from build123d import *

# Parameters (mm, degrees)
F0_W     = 114.3
F0_H     = 88.9
F1_DEPTH = 152.4
F3_R     = 38.1
F4_R     = 12.7
F5_DEPTH = 114.301
F6_R     = 6.35
F7_DEPTH = 38.1
F2_W     = 19.05
F2_H     = 88.9
F2_W_2   = 25.4
F8_DEPTH = 88.901


with BuildPart() as f1:
    # F0 (on Top) → F1 (new body)
    with BuildSketch(Plane.XY):
        Rectangle(F0_W, F0_H)
    extrude(amount=F1_DEPTH)

    # F3
    f3_edges = [f1.edges().sort_by_distance(p)[0] for p in [
        (0, -44.45, 152.4),
        (0, 44.45, 152.4),
    ]]
    fillet(f3_edges, radius=F3_R)

    # F4 (on face) → F5 (cut, through all)
    with BuildSketch(Plane(origin=(-57.15, 0, 0), x_dir=(0, -1, 0), z_dir=(-1, 0, 0))):
        with Locations((0, 38.1)):
            Circle(F4_R)
        with Locations((0, 114.3)):
            Circle(F4_R)
    extrude(amount=-F5_DEPTH, mode=Mode.SUBTRACT)

    # F6 (on face) → F7 (cut)
    with BuildSketch(Plane(origin=(0, 0, 0), x_dir=(1, 0, 0), z_dir=(0, 0, -1))):
        Circle(F6_R)
    extrude(amount=-F7_DEPTH, mode=Mode.SUBTRACT)

    # F2 (on face) → F8 (cut, through all)
    with BuildSketch(Plane.XZ.offset(44.45)):
        with Locations((-47.625, 107.95)):
            Rectangle(F2_W, F2_H)
        with Locations((0, 107.95)):
            Rectangle(F2_W_2, F2_H)
        with Locations((47.625, 107.95)):
            Rectangle(F2_W, F2_H)
    extrude(amount=-F8_DEPTH, mode=Mode.SUBTRACT)


solid = f1.part
Here's how the part is built. I have some questions about the finished solid (model axes, mm). A direction names the side the tool comes from. Coordinates: 2 decimals unless noted, no trailing zeros. Loops run counter-clockwise (first coordinate to the right, second up) from the corner with the lowest first, then second, coordinate; pieces in that order, holes last.
1. Imagine slicing it at B-B, the plane z = 38.1. Please give me the cut outline in (x, y), and give its area (3 significant figures).
2. I need wall thicknesses on L1, parallel to Z at x = -35.5, y = 1; L2, parallel to X at y = -24.5, z = 141; L3, parallel to Y at x = 23, z = 114. Which ranges of each line are inside material? Lowest first, please.
3. For P1, Ø15, axis at x = 51.5, y = 19.5, coming from the +Z side; P2, Ø8, axis at x = -19.5, y = -17, coming from the +Z side; P3, Ø8, axis at y = -24.5, z = 82.5, coming from the -X side, each with a flat end and sliding along its axis, tell me the tip position at first contact or that it passes through.
4. Imagine slicing it at A-A, the plane y = 0. Please give me the cut outline in (x, z).
5. For faces 5 (the flat face through (-12.7, -1, 97)), 6 (the flat face through (-57.15, -1, 24)), 7 (the flat face through (47, -1, 63.5)), 8 (the cylindrical face through (6.057, -1.907, 13.361)), which set-ups out of +Z, -Z, +X, -X, +Y, -Y let a thin tool reach every point of the face, with its end or its side?
6. Imagine slicing it at C-C, the plane x = -25. Please give me the cut outline in (y, z).
7. Imagine slicing it at D-D, the plane x = 0. Please give me the cut outline in (y, z).
8. If we mould it in two halves opening along Z, with no side actions, what happens to faces 1 (the cylindrical face through (-25.58, 2.75, 101.9)), 2 (the cylindrical face through (25.58, -33.59, 140.94)), 3 (the cylindrical face through (25.22, 2.75, 101.9)), 4 (the flat face through (-38.1, -1, 97))? For each: pulls with the +Z half, pulls with the -Z half, needs draft (parallel to the pull), parting line crosses it, or undercut.
Taken from the geometry:
1. outline: (-57.15, -44.45) - (57.15, -44.45) - (57.15, -12.7) - (-57.15, -12.7) - close; (-57.15, 12.7) - (57.15, 12.7) - (57.15, 44.45) - (-57.15, 44.45) - close
1. area: 7,260 mm2
2. L1: z = 0 to 25.44, 50.76 to 101.64, 126.96 to 152.4
2. L2: x = -38.1 to -12.7, 12.7 to 38.1
2. L3: y = -44.45 to -12.7, 12.7 to 44.45
3. P1: stops at z = 63.5
3. P2: stops at z = 151.82
3. P3: stops at x = -38.1
4. outline: (-57.15, 0) - (-6.35, 0) - (-6.35, 25.4) - (-57.15, 25.4) - close; (-57.15, 50.8) - (57.15, 50.8) - (57.15, 63.5) - (38.1, 63.5) - (38.1, 101.6) - (12.7, 101.6) - (12.7, 63.5) - (-12.7, 63.5) - (-12.7, 101.6) - (-38.1, 101.6) - (-38.1, 63.5) - (-57.15, 63.5) - close; (-38.1, 127) - (-12.7, 127) - (-12.7, 152.4) - (-38.1, 152.4) - close; (6.35, 0) - (57.15, 0) - (57.15, 25.4) - (6.35, 25.4) - close; (12.7, 127) - (38.1, 127) - (38.1, 152.4) - (12.7, 152.4) - close
5. face 5: +Z, +Y, -Y
5. face 6: +Z, -Z, -X, +Y, -Y
5. face 7: +Z, +X, +Y, -Y
5. face 8: -Z
6. outline: (-44.45, 0) - (44.45, 0) - (44.45, 114.3) arc R38.1 ccw to (6.35, 152.4) - (-6.35, 152.4) arc R38.1 ccw to (-44.45, 114.3) - close; hole circle Ø25.4 at (0, 38.1); hole circle Ø25.4 at (0, 114.3)
7. outline: (-44.45, 0) - (-6.35, 0) - (-6.35, 27.1) arc R12.7 cw (long way) to (6.35, 27.1) - (6.35, 0) - (44.45, 0) - (44.45, 63.5) - (-44.45, 63.5) - close
8. face 1: undercut
8. face 2: pulls with the +Z half
8. face 3: undercut
8. face 4: needs draft
